The model under review builds one solid part; all positions refer to its coordinate system, in mm. A direction names the side the tool comes from. Coordinates: 2 decimals unless noted, no trailing zeros. Loops run counter-clockwise (first coordinate to the right, second up) from the corner with the lowest first, then second, coordinate; pieces in that order, holes last. Notation, with made-up numbers: (88, -32) - (109, -32) arc R25 ccw to (109, 1) - close; hole circle Ø3 at (-0.5, -23). An arc over 180 degrees is marked (long way). Use a Markdown table: item, result. Add a question column.
1) For faces 1 (the flat face through (-43.188, -43, 49)), 2 (the flat face through (0, -96, 49)), list the 3-axis set-ups (+Z, -Z, +X, -X, +Y, -Y) from which the entire face can be reached by the end or side of a thin tool; tool diameter is ignored.
2) Add section D-D, the plane z = 37. Give the boundary of the cut face in (x, y).
3) Add section B-B, the plane z = 50. Give the boundary of the cut face in (x, y).
4) Add section C-C, the plane x = -15.5. Give the boundary of the cut face in (y, z).
5) Add section A-A, the plane y = -59. Give the boundary of the cut face in (x, z), and give its area (3 significant figures).
6) To check wall thickness, follow L1, parallel to X at y = -17.5, z = 22; L2, parallel to Y at x = 2, z = 91.5; L3, parallel to X at y = -90.5, z = 23.5. State the ranges of each line that lie inside material, in increasing order. Write a range as [from, to].
7) Clearance check with flat-ended pins moving along their axes: pin 1 (2 mm diameter, centred on x = -36.5, z = 71, fed in from +Y); pin 2 (6 mm diameter, centred on x = 9.5, z = 43.5, fed in from +Y). State where each tip first meets the part, or that it passes through.
8) The part is to be moulded in two halves that separate along Z. For faces 3 (the cylindrical face through (-44.17, -11.49, 47.69)), 4 (the flat face through (0, -94, 100)), 5 (the flat face through (-38.79, -88.4, 49.3)), say which applies: pulls with the +Z half, pulls with the -Z half, needs draft (parallel to the pull), parting line crosses it, or undercut.
Autodesk Inventor part; units mm, degrees
ref_plane "YZ Plane" through (0, 0, 0) normal (1, 0, 0) x (0, 1, 0)
ref_plane "XZ Plane" through (0, 0, 0) normal (0, 1, 0) x (-1, 0, 0)
ref_plane "XY Plane" through (0, 0, 0) normal (0, 0, 1) x (1, 0, 0)
sketch "Sketch1" plane through (0, 0, 0) normal (0, 0, 1) x (1, 0, 0)
  line L0 (-46.188, 0) -> (-23.094, 40)
  line L1 (-23.094, 40) -> (23.094, 40)
  line L2 (23.094, 40) -> (46.188, 0)
  line L3 (46.188, 0) -> (23.094, -40)
  line L4 (23.094, -40) -> (-23.094, -40)
  line L5 (-23.094, -40) -> (-46.188, 0)
  line L6 (-48.188, 0) -> (-46.188, 0)
  line L7 (46.188, 0) -> (48.188, 0)
  line L8 (-46.188, 0) -> (-43.188, -5.1962)
  line L9 (46.188, 0) -> (43.188, -5.1962)
  line L10 (-46.188, 0) -> (-46.188, -81)
  line L11 (-46.188, -81) -> (-31.188, -96)
  line L12 (-31.188, -96) -> (31.188, -96)
  line L13 (31.188, -96) -> (46.188, -81)
  line L14 (46.188, -81) -> (46.188, 0)
  line L15 (43.188, -5.1962) -> (43.188, -79.7574)
  line L16 (43.188, -79.7574) -> (29.9454, -93)
  line L17 (29.9454, -93) -> (-29.9454, -93)
  line L18 (-29.9454, -93) -> (-43.188, -79.7574)
  line L19 (-43.188, -79.7574) -> (-43.188, -5.1962)
  point P0 (0, 0)
  point P1 (0, 0)
  point P2 (0, -96)
  dimension "d0" = 80
  dimension "d6" = 56
  dimension "d7" = 15
  dimension "d8" = 15
  dimension "d9" = 3
extrude "Extrusion1" add sketch "Sketch1" along normal blind 100 contours L5 L19 L18 L17 L16 L15 L3 L14 L13 L12 L11 L10
sketch "Sketch2" plane through (-46.188, 0, 100) normal (0.866, 0.5, 0) x (0, 0, -1)
  circle A0 centre (50, -10) radius 2.5
  line L0 (100, 0) -> (0, 0)
  point P0 (100, -23.094)
  point P1 (50, 0)
  dimension "d10" = 5
  dimension "d11" = 10
extrude "Extrusion2" cut sketch "Sketch2" against normal through all
sketch "Sketch3" plane through (43.188, -5.1962, 0) normal (-0.866, 0.5, 0) x (0, 0, 1)
  circle A0 centre (50, -4) radius 2.5
  line L0 (0, 6) -> (100, 6)
  point P0 (0, -17.094)
  point P1 (50, 6)
  dimension "d14" = 5
  dimension "d15" = 10
extrude "Extrusion3" cut sketch "Sketch3" against normal through all
properties part number "A03" material "ABS Plastic"
From the geometry:
| question | item | result |
|---|---|---|
| 1 | face 1 | +Z, -Z, +Y |
| 1 | face 2 | +Z, -Z, +X, -X, -Y |
| 2 | outline | (-46.19, -81) - (-31.19, -96) - (31.19, -96) - (46.19, -81) - (46.19, 0) - (43.19, -5.2) - (43.19, -79.76) - (29.95, -93) - (-29.95, -93) - (-43.19, -79.76) - (-43.19, -5.2) - (-46.19, 0) - close |
| 3 | outline | (-46.19, -81) - (-31.19, -96) - (31.19, -96) - (46.19, -81) - (46.19, -14.43) - (43.19, -12.7) - (43.19, -79.76) - (29.95, -93) - (-29.95, -93) - (-43.19, -79.76) - (-43.19, -12.7) - (-46.19, -14.43) - close; (-46.19, -8.66) - (-43.19, -6.93) - (-43.19, -5.2) - (-46.19, 0) - close; (43.19, -6.93) - (46.19, -8.66) - (46.19, 0) - (43.19, -5.2) - close |
| 4 | outline | (-96, 0) - (-93, 0) - (-93, 100) - (-96, 100) - close |
| 5 | outline | (-46.19, 0) - (-43.19, 0) - (-43.19, 100) - (-46.19, 100) - close; (43.19, 0) - (46.19, 0) - (46.19, 100) - (43.19, 100) - close |
| 5 | area | 600 mm^2 |
| 6 | L1 | x = [-46.19, -43.19], [43.19, 46.19] |
| 6 | L2 | y = [-96, -93] |
| 6 | L3 | x = [-36.69, -32.45], [32.45, 36.69] |
| 7 | pin 1 | stops at y = -85.45 |
| 7 | pin 2 | stops at y = -93 |
| 8 | face 3 | undercut |
| 8 | face 4 | pulls with the +Z half |
| 8 | face 5 | needs draft |
